Geometry: see drawing. Coordinates: mm, zero at the bounding-box minimum. Coordinates: 2 decimals unless noted, no trailing zeros. Order: outer loops, then holes, each group sorted by start corner. A loop starts at its lowest first (then second) coordinate and runs counter-clockwise, first axis right, second up.
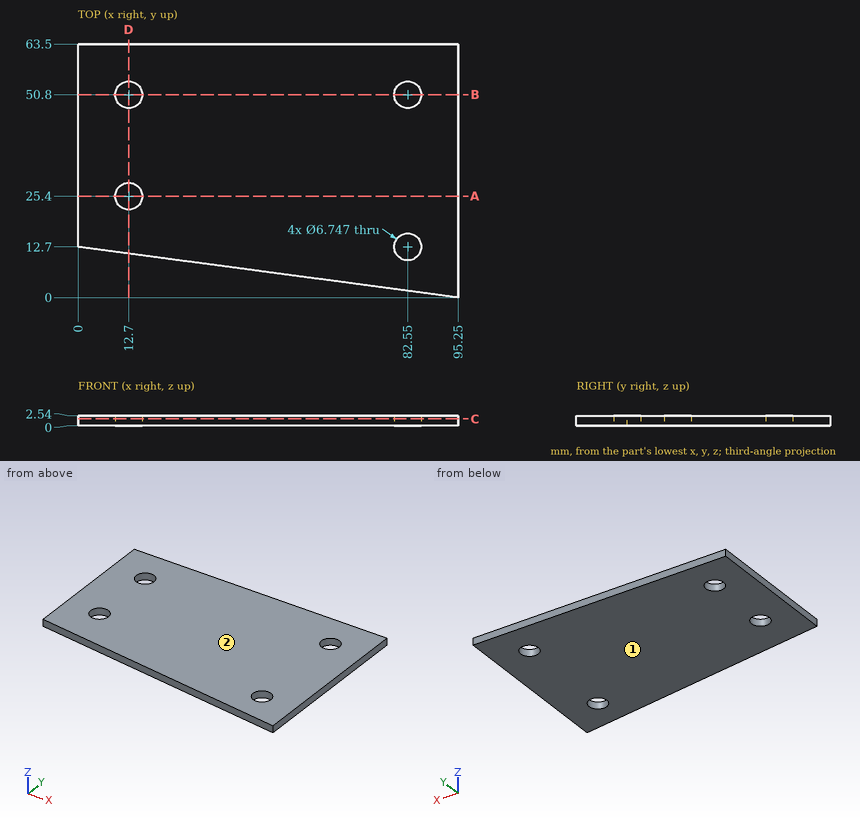
Q1. Pin query (flat end, axial travel): P1, Ø4, axis at x = 82.55, y = 50.8, coming from the +Z side. Return the tip coordinate at first contact, or that it passes through.
Solutions:
P1: passes through
Q2. Section query D-D on x = 12.7. Output: boundary loops of the cut face in (y, z).
Solutions:
outline: (11.01, 0) - (22.03, 0) - (22.03, 2.54) - (11.01, 2.54) - close; (28.77, 0) - (47.43, 0) - (47.43, 2.54) - (28.77, 2.54) - close; (54.17, 0) - (63.5, 0) - (63.5, 2.54) - (54.17, 2.54) - close
Q3. Section query A-A on y = 25.4. Output: boundary loops of the cut face in (x, z), plus the area to 3 significant figures.
Solutions:
outline: (0, 0) - (9.33, 0) - (9.33, 2.54) - (0, 2.54) - close; (16.07, 0) - (95.25, 0) - (95.25, 2.54) - (16.07, 2.54) - close
area: 225 mm2
Q4. Pull-direction query (Z, two-part tool) for the marked faces 1 and 2; classes: pulls with the +Z half, pulls with the -Z half, needs draft (parallel to the pull), parting line crosses it, or undercut.
Solutions:
face 1: pulls with the -Z half
face 2: pulls with the +Z half
Q5. Material intervals for line 1 along Y through (x, z) = (12.7, 2.05); line 2 along X through (y, z) = (23, 0.75); line 3 along Y through (x, z) = (82.55, 1.9), sorted ascending.
Solutions:
line 1: y = 11.01 to 22.03, 28.77 to 47.43, 54.17 to 63.5
line 2: x = 0 to 10.33, 15.07 to 95.25
line 3: y = 1.69 to 9.33, 16.07 to 47.43, 54.17 to 63.5
Q6. Section query B-B on y = 50.8. Output: boundary loops of the cut face in (x, z).
Solutions:
outline: (0, 0) - (9.33, 0) - (9.33, 2.54) - (0, 2.54) - close; (16.07, 0) - (79.18, 0) - (79.18, 2.54) - (16.07, 2.54) - close; (85.92, 0) - (95.25, 0) - (95.25, 2.54) - (85.92, 2.54) - close
Q7. Section query C-C on z = 1.7. Output: boundary loops of the cut face in (x, y).
Solutions:
outline: (0, 12.7) - (95.25, 0) - (95.25, 63.5) - (0, 63.5) - close; hole circle Ø6.75 at (12.7, 25.4); hole circle Ø6.75 at (12.7, 50.8); hole circle Ø6.75 at (82.55, 12.7); hole circle Ø6.75 at (82.55, 50.8)
